Can you work these out from the drawing? Everything is in mm from the part's minimum corner. A direction names the side the tool comes from. Coordinates: 2 decimals unless noted, no trailing zeros. Loops run counter-clockwise (first coordinate to the right, second up) from the corner with the lowest first, then second, coordinate; pieces in that order, holes last.
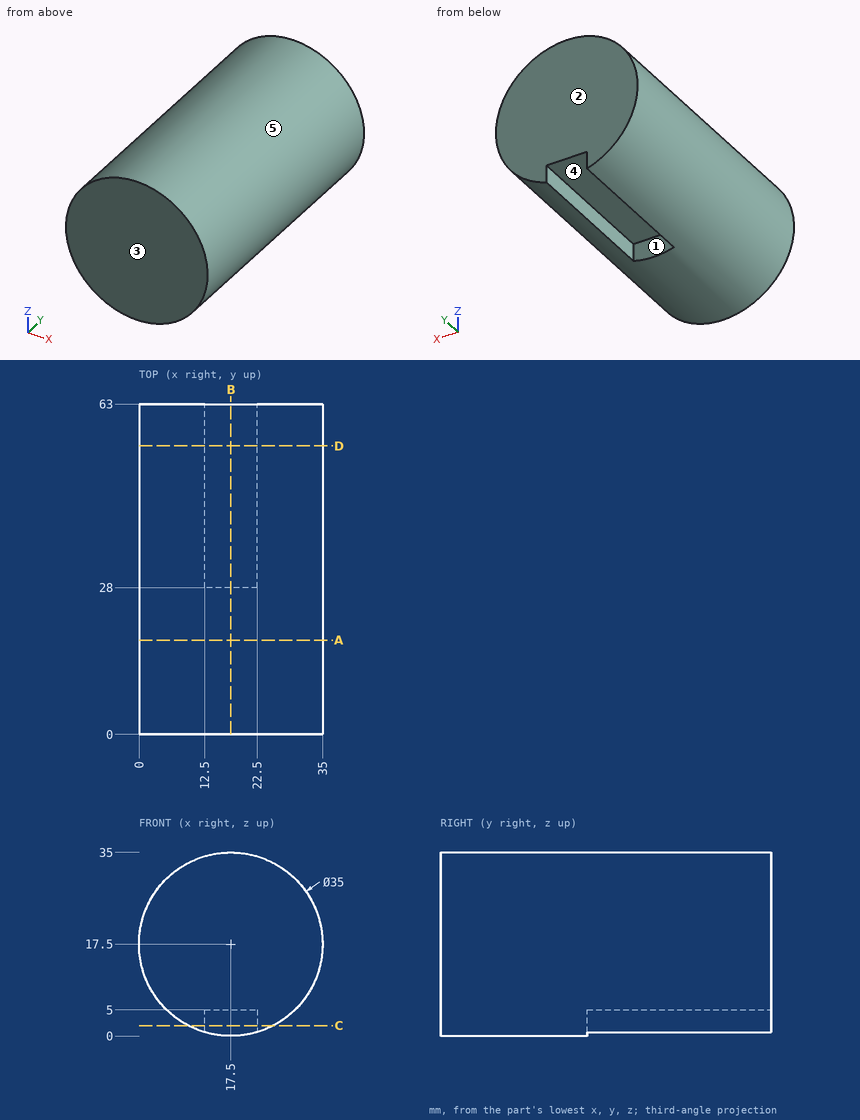
1. I want a section at D-D (y = 55). Please give me the cut outline in (x, z).
2. We'd pull the mould along X, two halves only. Please class the marked faces 3, 4 and 5: +X half, -X half, draft (parallel to the pull), parting line (faces both ways), or undercut.
3. For pin 1 (10 mm diameter, centred on y = 11, z = 6, fed in from +X); pin 2 (1 mm diameter, centred on x = 14.5, y = 46.5, fed in from +Z); pin 3 (1.3 mm diameter, centred on y = 38.5, z = 3, fed in from +X), each with a flat end and sliding along its axis, tell me the tip position at first contact or that it passes through.
4. I want a section at A-A (y = 18). Please give me the cut outline in (x, z).
5. On a 3-axis mill with a long thin cutter (end or side, diameter ignored), from which of +Z, -Z, +X, -X, +Y, -Y can I reach the whole of each face in a straight line? I mean the marked faces 1 and 2. Say none if no direction works.
6. I want a section at B-B (x = 17.5). Please give me the cut outline in (y, z).
7. I need wall thicknesses on line 1 along X through (y, z) = (10.5, 18); line 2 along Z through (x, y) = (17.5, 47); line 3 along X through (y, z) = (35, 3). Which ranges of each line are inside material? Lowest first, please.
8. I want a section at C-C (z = 2). Please give me the cut outline in (x, y).
Response values:
1. outline: (12.5, 0.73) - (12.5, 5) - (22.5, 5) - (22.5, 0.73) arc R17.5 ccw (long way) to start
2. face 3: draft
2. face 4: undercut
2. face 5: parting line
3. pin 1: stops at x = 33.75
3. pin 2: stops at z = 34.82
3. pin 3: stops at x = 28.2
4. outline: circle Ø35 at (17.5, 17.5)
5. face 1: -Z, +Y
5. face 2: +Z, -Z, +X, -X, +Y
6. outline: (0, 0) - (28, 0) - (28, 5) - (63, 5) - (63, 35) - (0, 35) - close
7. line 1: x = 0.01 to 34.99
7. line 2: z = 5 to 35
7. line 3: x = 7.7 to 12.5, 22.5 to 27.3
8. outline: (9.38, 0) - (25.62, 0) - (25.62, 63) - (22.5, 63) - (22.5, 28) - (12.5, 28) - (12.5, 63) - (9.38, 63) - close
